Read the model definition and answer for the solid it produces. Units are mm, in the model's axes. A direction names the side the tool comes from. Give positions to 0.01 mm unless a question says otherwise; leave off trailing zeros. Write each loop counter-clockwise with the first axis right and the second up, starting at its lowest first coordinate (ties: lowest second). Pieces come first, ordered by that corner, then holes. Notation, with made-up numbers: M -30,64.25 L 27,64.25 A27 ccw 27,101.25 Z; hole C 79,49.5 d10. An arc over 180 degrees is marked long. Put each result on its own line as item: value.
from build123d import *

# Parameters (mm, degrees)
RESSALTO_EXTRUS_O1_DEPTH   = 4
ESBO_O2_R                  = 1
CORTE_EXTRUS_O1_DEPTH      = 227.530351
CORTE_EXTRUS_O2_DEPTH      = 186.712143
CORTE_EXTRUS_O2_DEPTH_BACK = 186.712143
ESBO_O3_R                  = 1.5


with BuildPart() as part:
    # Esboço1 → Ressalto-extrusão1 (new body)
    with BuildSketch(Plane(origin=(0, 0, 0), x_dir=(1, 0, 0), z_dir=(0, 1, 0))):
        Polygon((90, -51.961524), (90, 51.961524), (0, 103.923048), (-90, 51.961524), (-90, -51.961524), (0, -103.923048), align=None)
        Polygon((87, 50.229473), (0, 100.458947), (-87, 50.229473), (-87, -50.229473), (0, -100.458947), (87, -50.229473), align=None, mode=Mode.SUBTRACT)
    extrude(amount=RESSALTO_EXTRUS_O1_DEPTH)

    # Esboço2 → Corte-extrusão1 (cut, through all)
    with BuildSketch(Plane(origin=(-45, 0, 77.942286), x_dir=(0.8660254037844387, 0, 0.49999999999999994), z_dir=(-0.4999999999999999, 0, 0.8660254037844386))):
        with Locations((0, 2)):
            Circle(ESBO_O2_R)
    extrude(amount=-CORTE_EXTRUS_O1_DEPTH, mode=Mode.SUBTRACT)

    # Esboço3 → Corte-extrusão2 (cut, two sides: drawn at the far end of the back side and taken through both)
    with BuildSketch(Plane(origin=(-43.5, 0, -25.114737), x_dir=(-0.5, 0, 0.8660254037844386), z_dir=(-0.8660254037844387, 0, -0.5000000000000001)).offset(-CORTE_EXTRUS_O2_DEPTH_BACK)):
        with Locations(Location((0, 2, 0), (0, 0, 90))):
            Circle(ESBO_O3_R)
    extrude(amount=CORTE_EXTRUS_O2_DEPTH + CORTE_EXTRUS_O2_DEPTH_BACK, mode=Mode.SUBTRACT)


solid = part.part
(1) Section B-B on x = -25.5 is taken. Determine the outline of the cut face in (y, z), and give its area (3 significant figures).
Result:
outline: M 0,-89.2 L 4,-89.2 L 4,-85.74 L 0,-85.74 Z; M 0,85.74 L 4,85.74 L 4,89.2 L 0,89.2 Z
area: 27.7 mm²
(2) For a pull along X with two mould halves and no side action, classify faces 1 (the face through (-44.37, 1.972, -78.306)), 2 (the face through (45.63, 1.08, -77.58)), 3 (the face through (-44.11, 1.08, 74.99)) as +X half, -X half, draft (parallel to the pull), parting line (faces both ways), or undercut.
Result:
face 1: -X half
face 2: +X half
face 3: undercut
(3) Straight lines are drawn through the part: line 1 along X through (y, z) = (2.4, -20); line 2 along Z through (x, y) = (8, 3.3); line 3 along Z through (x, y) = (-69.5, 1.4). For each, find the intervals that lie inside material, in ascending order. Write a range as from..to.
Result:
line 1: x = -90..-87, 87..90
line 2: z = -99.3..-95.84, 95.84..99.3
line 3: z = -63.8..-60.33, 60.33..63.8
(4) Given pin 1 Ø2 at (y, z) = (0.5, 75.5) entering from -X, flat-ended and moving along its own axis, determine where the tip first touches the part or whether it passes through.
Result:
pin 1: stops at x = -50.96
(5) Which of the six approach directions +Z, -Z, +X, -X, +Y, -Y give full straight-line access (tool end or side, diameter ignored) to faces 4 (the face through (-42.891, 1.972, -75.696)), 5 (the face through (87.38, 1.67, 52.14))?
Result:
face 4: +Y, -Y
face 5: none
(6) Section A-A on z = 65.5 is taken. Determine the outline of the cut face in (x, y), and give its area (3 significant figures).
Result:
outline: M -66.55,0 L -60.55,0 L -60.55,4 L -66.55,4 Z; M 60.55,0 L 66.55,0 L 66.55,4 L 60.55,4 Z
area: 48.0 mm²
